Print and shaded views of the part. All mm, measured from the part's lowest x, y and z. Give positions to 0.01 mm unless a question says otherwise; leave off trailing zeros. Loops run counter-clockwise (first coordinate to the right, second up) from the corner with the lowest first, then second, coordinate; pieces in that order, holes last.
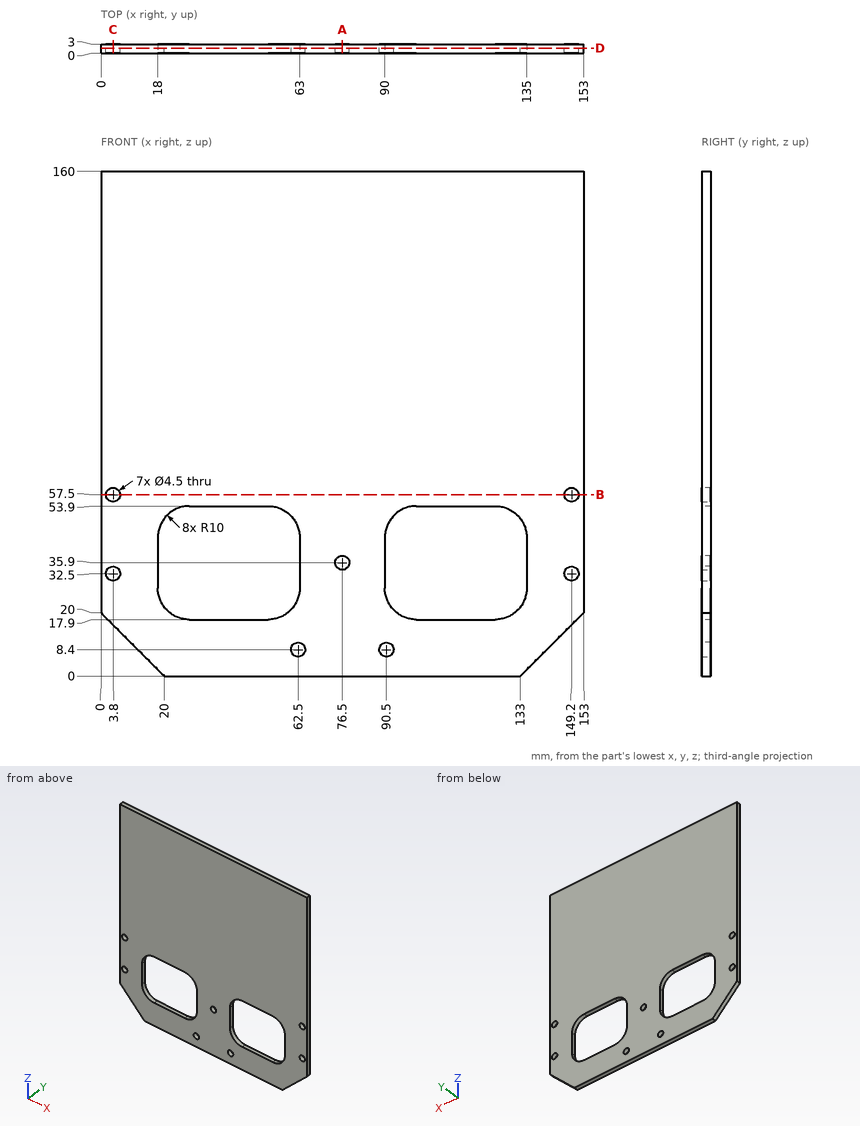
1. Saw through at C-C, the plane x = 3.8. List the corners of the cut face in (y, z), and give its area (3 significant figures).
Responses:
outline: (0, 16.2) - (3, 16.2) - (3, 30.25) - (0, 30.25) - close; (0, 34.75) - (3, 34.75) - (3, 55.25) - (0, 55.25) - close; (0, 59.75) - (3, 59.75) - (3, 160) - (0, 160) - close
area: 404 mm2
2. Saw through at B-B, the plane z = 57.5. List the corners of the cut face in (x, y).
Responses:
outline: (0, 0) - (1.55, 0) - (1.55, 3) - (0, 3) - close; (6.05, 0) - (146.95, 0) - (146.95, 3) - (6.05, 3) - close; (151.45, 0) - (153, 0) - (153, 3) - (151.45, 3) - close
3. Saw through at D-D, the plane y = 1.7. Count the separate pieces of the cut face and the enclosed holes in it, and give its area (3 significant figures).
Responses:
separate pieces: 1
enclosed holes: 9
area: 20,900 mm2
4. Saw through at A-A, the plane x = 76.5. List the corners of the cut face in (y, z), and give its area (4 significant figures).
Responses:
outline: (0, 0) - (3, 0) - (3, 33.65) - (0, 33.65) - close; (0, 38.15) - (3, 38.15) - (3, 160) - (0, 160) - close
area: 466.5 mm2
5. Probe line 1 along X through (y, z) = (1.1, 32.5); line 2 along X through (y, z) = (1.55, 35.9); line 3 along X through (y, z) = (1.85, 8.4). List the from-to ranges inside material, lowest first.
Responses:
line 1: x = 0 to 1.55, 6.05 to 18, 63 to 90, 135 to 146.95, 151.45 to 153
line 2: x = 0 to 18, 63 to 74.25, 78.75 to 90, 135 to 153
line 3: x = 11.6 to 60.25, 64.75 to 88.25, 92.75 to 141.4
